Here's how the part is built. I have some questions about the finished solid (model axes, mm). A direction names the side the tool comes from. Give positions to 0.01 mm unless a question says otherwise; leave off trailing zeros. Write each loop counter-clockwise with the first axis right and the second up, starting at its lowest first coordinate (ties: lowest second). Pieces come first, ordered by that corner, then holes. Notation, with made-up numbers: (35, 28) -> (50, 28) arc R21 ccw to (50, 45) -> close; hole circle Ø5 at (72, 87.5). An arc over 180 degrees is marked (long way). Use one line per item in the form item = value.
```python
from build123d import *

# Parameters (mm, degrees)
BOSS_EXTRUDE1_DEPTH      = 7
BOSS_EXTRUDE2_DEPTH      = 13
BOSS_EXTRUDE2_DEPTH_BACK = 20
SKETCH2_W                = 5
SKETCH2_H                = 10
SKETCH4_R                = 2.1
CUT_EXTRUDE1_DEPTH       = 78.679302724
FILLET1_R                = 1


with BuildPart() as part:
    # Sketch1 → Boss-Extrude1 (new body)
    with BuildSketch(Plane.YZ):
        Polygon((0, 0), (-5, 0), (-5, 10), (0, 10), (0, 8.5), (12.487376862, 8.5), (36.687835728, -60.999037426), (37.088615702, -62.15), (29.67637193, -62.15), (7.512623138, 1.5), (0, 1.5), align=None)
    extrude(amount=BOSS_EXTRUDE1_DEPTH)

    # Sketch2 → Boss-Extrude2 (add, two sides: drawn at the far end of the back side and taken through both)
    with BuildSketch(Plane.YZ.offset(7).offset(-BOSS_EXTRUDE2_DEPTH_BACK)):
        with Locations((-2.5, 5)):
            Rectangle(SKETCH2_W, SKETCH2_H)
    extrude(amount=BOSS_EXTRUDE2_DEPTH + BOSS_EXTRUDE2_DEPTH_BACK)

    # Sketch4 → Cut-Extrude1 (cut, through all)
    with BuildSketch(Plane.XZ.offset(5)):
        with Locations(Location((-6.5, 5, 0), (0, 0, 270))):
            Circle(SKETCH4_R)
        with Locations(Location((13.5, 5, 0), (0, 0, 270))):
            Circle(SKETCH4_R)
    extrude(amount=-CUT_EXTRUDE1_DEPTH, mode=Mode.SUBTRACT)

    # Fillet1
    fillet1_edges = [part.edges().sort_by_distance(p)[0] for p in [
        (0, 6.243688431, 8.5),
        (0, 24.787996282, -26.825),
        (0, 18.594497534, -30.325),
        (0, 3.756311569, 1.5),
        (3.5, 12.487376862, 8.5),
        (3.5, 0, 0),
        (3.5, -5, 10),
        (3.5, 0, 10),
        (7, 3.756311569, 1.5),
        (7, 18.594497534, -30.325),
        (-13, -2.5, 10),
        (7, 24.787996282, -26.825),
        (-13, 0, 5),
        (-13, -2.5, 0),
        (20, -2.5, 0),
        (20, 0, 5),
        (20, -2.5, 10),
        (7, 6.243688431, 8.5),
    ]]
    fillet(fillet1_edges, radius=FILLET1_R)


solid = part.part
```
Q1. I want a section at D-D, the plane z = 5. Count the separate pieces of the cut face and the enclosed holes in it, and give its area (3 significant figures).
Result set:
separate_pieces = 3
enclosed_holes = 0
area = 218 mm2
Q2. I want a section at C-C, the plane x = -2. Write out the boundary of the cut face in (y, z), and give its area (3 significant figures).
Result set:
outline = (-5, 0) -> (-1, 0) arc R1 ccw to (0, 1) -> (0, 9) arc R1 ccw to (-1, 10) -> (-4, 10) arc R1 ccw to (-5, 9) -> close
area = 49.4 mm2
Q3. Will these pins go through, and if not, where does the flat tip stop? pin 1 Ø6 at (x, y) = (7.5, 11) entering from +Z; pin 2 Ø9 at (x, z) = (4, 4) entering from +Y; pin 3 Ø12 at (y, z) = (12, 2.5) entering from +X.
Result set:
pin_1 = 8.5
pin_2 = 15.62
pin_3 = 7
Q4. I want a section at A-A, the plane x = 13.5. Write out the boundary of the cut face in (y, z), and give its area (3 significant figures).
Result set:
outline = (-5, 0) -> (-1, 0) arc R1 ccw to (0, 1) -> (0, 2.9) -> (-5, 2.9) -> close; (-5, 7.1) -> (0, 7.1) -> (0, 9) arc R1 ccw to (-1, 10) -> (-4, 10) arc R1 ccw to (-5, 9) -> close
area = 28.4 mm2
Q5. Which directions (+Z, -Z, +X, -X, +Y, -Y) give clear straight access to the entire face, cutting with the end or side of a thin tool? Please do faces 4 (the face through (7, 19, -25)), 5 (the face through (3, -3, 0)), 6 (the face through (3, 4, 1.5)), 7 (the face through (3, 6, 8.5)).
Result set:
face_4 = +Z, -Z, +X, +Y
face_5 = -Z, +X, -X, -Y
face_6 = -Z, +X, -X
face_7 = +Z, +X, -X, +Y
Q6. If I drill on line 1 along X through (y, z) = (-1.2, 5); line 2 along X through (y, z) = (31, -57.5); line 3 along Y through (x, z) = (0.5, -40), over which ranges is the centre line in solid material (lowest first)? Write a range as from..to.
Result set:
line_1 = -13..-8.6, -4.4..11.4, 15.6..20
line_2 = 0..7
line_3 = 22.11..29.23
Q7. I want a section at B-B, the plane y = 2.5. Write out the boundary of the cut face in (x, z).
Result set:
outline = (0, 2.5) arc R1 ccw to (1, 1.5) -> (6, 1.5) arc R1 ccw to (7, 2.5) -> (7, 7.5) arc R1 ccw to (6, 8.5) -> (1, 8.5) arc R1 ccw to (0, 7.5) -> close
Q8. If we mould it in two halves opening along Z, with no side actions, what happens to faces 1 (the face through (0.285, 18.661, -29.602)), 2 (the face through (0, 19, -25)), 3 (the face through (-4.418, -2.535, 5.273))? For each: +Z half, -Z half, draft (parallel to the pull), parting line (faces both ways), or undercut.
Result set:
face_1 = -Z half
face_2 = draft
face_3 = undercut
